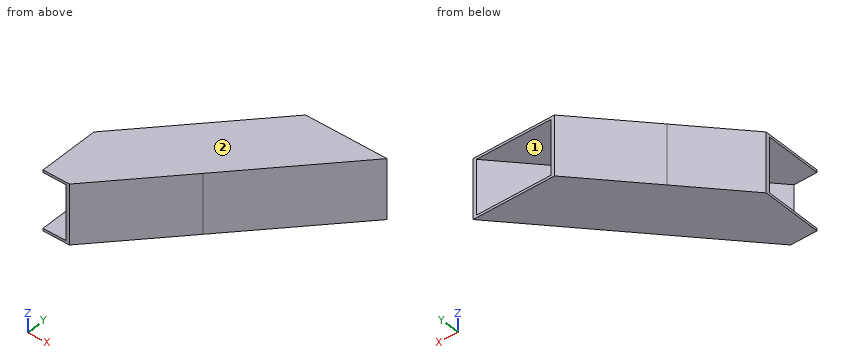
```python
from build123d import *

# Parameters (mm, degrees)
BOSS_EXTRUDE1_DEPTH = 38.1
SHELL1_T            = -3.175
CUT_EXTRUDE6_DEPTH  = 76.2


with BuildPart() as part:
    # Sketch2 → Boss-Extrude1 (new, symmetric)
    with BuildSketch(Plane.XY):
        Polygon((46.237705824, 106.855650642), (-28.090411256, 25.739828971), (28.090411256, -25.739828971), (149.590411256, 106.855650642), align=None)
        Polygon((-28.090411256, 25.739828971), (-93.409588744, -45.544349358), (-93.409588744, -158.335308585), (28.090411256, -25.739828971), align=None)
    extrude(amount=BOSS_EXTRUDE1_DEPTH, both=True)

    # Shell1
    shell1_openings = [part.faces().sort_by_distance(p)[0] for p in [
        (97.91405854, 106.855650642, 0),
        (-93.409588744, -101.939828971, 0),
    ]]
    offset(amount=SHELL1_T, openings=shell1_openings, kind=Kind.INTERSECTION)

    # Sketch3 → Cut-Extrude6 (cut)
    with BuildSketch(Plane.XY.offset(38.1)):
        Polygon((-59.880530596, -121.744349358), (-93.409588744, -121.744349358), (-93.409588744, -158.335308585), align=None)
    extrude(amount=-CUT_EXTRUDE6_DEPTH, mode=Mode.SUBTRACT)


solid = part.part
```
Input: part model. Units: mm. Frame: model coordinates. Face numbers are marked on the shaded views. Coordinates: 2 decimals unless noted, no trailing zeros. Loops run counter-clockwise (first coordinate to the right, second up) from the corner with the lowest first, then second, coordinate; pieces in that order, holes last. Notation, with made-up numbers: M -12.75,51.25 L 19.25,51.25 A25 cw 19.25,73.25 Z; hole C -39,42.25 d4. An arc over 180 degrees is marked long. Use a Markdown table: item, result. Add a question column.
1) Pin query (flat end, axial travel): P1, Ø10, axis at y = 31, z = -24.5, coming from the -X side; P2, Ø1, axis at x = 49.5, z = -22, coming from the -Y side; P3, Ø10, axis at x = 90.5, z = 20, coming from the +Y side. Return the tip coordinate at first contact, or that it passes through.
2) Section A-A, the plane z = 2.5. Return the cut outline in (x, y), plus the area to 3 significant figures.
3) Draft query along Y for the marked faces 1 and 2. Return one class per face: +Y half, -Y half, draft (parallel to the pull), parting line (faces both ways), or undercut.
4) Line query: L1, parallel to Z at x = -60, y = -98 (3 decimals); L2, parallel to X at y = 12.5, z = -9; L3, parallel to Y at x = -44, z = -17. Output: solid intervals per line, ascending. Write a range as from..to.
5) Section B-B, the plane x = 96. Return the cut outline in (y, z) (3 decimals).
6) Section C-C, the plane y = 17.5. Return the cut outline in (x, z) (3 decimals).
7) Section D-D, the plane x = -9.5. Return the cut outline in (y, z) (3 decimals).
Answer below:
| question | item | result |
|---|---|---|
| 1 | P1 | x = -27.85 |
| 1 | P2 | y = -2.92 |
| 1 | P3 | y = 52.53 |
| 2 | outline | M -93.41,-50.24 L 50.54,106.86 L 46.24,106.86 L -93.41,-45.54 Z; M -64.19,-121.74 L -59.88,-121.74 L 149.59,106.86 L 145.28,106.86 Z |
| 2 | area | 1,650 mm2 |
| 3 | face 1 | undercut |
| 3 | face 2 | draft |
| 4 | L1 | -38.1..-34.925, 34.925..38.1 |
| 4 | L2 | -40.22..-35.92, 58.82..63.13 |
| 4 | L3 | -104.41..-99.71, 3.68..8.38 |
| 5 | outline | M 48.371,-38.1 L 106.856,-38.1 L 106.856,-34.925 L 53.071,-34.925 L 53.071,34.925 L 106.856,34.925 L 106.856,38.1 L 48.371,38.1 Z |
| 6 | outline | M -35.641,-38.1 L 67.712,-38.1 L 67.712,38.1 L -35.641,38.1 Z; hole M -31.334,-34.925 L 63.406,-34.925 L 63.406,34.925 L -31.334,34.925 Z |
| 7 | outline | M -66.763,-38.1 L 46.028,-38.1 L 46.028,38.1 L -66.763,38.1 Z; hole M -62.063,-34.925 L 41.328,-34.925 L 41.328,34.925 L -62.063,34.925 Z |
